from build123d import *

# Parameters (mm, degrees)
BOSS_EXTRU_1_DEPTH      = 6
BOSS_EXTRU_2_DEPTH      = 1.25
BOSS_EXTRU_2_DEPTH_BACK = 1.25
BOSS_EXTRU_3_DEPTH      = 1
ESQUISSE4_W             = 9.998484941
ESQUISSE4_H             = 1.4
BOSS_EXTRU_4_DEPTH      = 4.5
ESQUISSE6_W             = 1.25
ESQUISSE6_H             = 4.5
ENL_V_MAT_EXTRU_1_DEPTH = 0.7
CHANFREIN1_SIZE         = 0.7
BOSS_EXTRU_5_DEPTH      = 1.351515059
BOSS_EXTRU_6_DEPTH      = 1.35
ESQUISSE9_W             = 0.76
ESQUISSE9_H             = 0.76
BOSS_EXTRU_7_DEPTH      = 4
CHANFREIN2_SIZE         = 0.25
ENL_V_MAT_EXTRU_2_REACH = 11.014
ESQUISSE10_W            = 5
ESQUISSE10_H            = 3.75
CHANFREIN3_SIZE         = 0.25
ENL_V_MAT_EXTRU_3_REACH = 11.274
ESQUISSE11_W            = 5
ESQUISSE11_H            = 1.25


with BuildPart() as part:
    # Esquisse1 → Boss.-Extru.1 (new body)
    with BuildSketch(Plane.XY):
        Polygon((5, 0), (-5, 0), (-5, 5.5), (-3.33, 5.5), (-3.33, 4.5), (3.33, 4.5), (3.33, 5.5), (5, 5.5), align=None)
        Polygon((-4.5, 5), (-3.53, 5), (-3.53, 4), (3.53, 4), (3.53, 5), (4.5, 5), (4.5, 0.5), (-4.5, 0.5), align=None, mode=Mode.SUBTRACT)
    extrude(amount=BOSS_EXTRU_1_DEPTH)

    # Esquisse2 → Boss.-Extru.2 (add, two sides: drawn at the far end of the back side and taken through both)
    with BuildSketch(Plane(origin=(0, 0, 0), x_dir=(0, 0, -1), z_dir=(1, 0, 0)).offset(-BOSS_EXTRU_2_DEPTH_BACK)):
        Polygon((-1, 5.5), (-2.5, 4.5), (-0.9, 4.5), (-0.9, 5.5), align=None)
    extrude(amount=BOSS_EXTRU_2_DEPTH + BOSS_EXTRU_2_DEPTH_BACK)

    # Esquisse3 → Boss.-Extru.3 (add)
    with BuildSketch(Plane(origin=(0, 0, 0), x_dir=(-1, 0, 0), z_dir=(0, 0, -1))):
        Polygon((-3.33, 5.5), (-5, 5.5), (-5, 0), (5, 0), (5, 5.5), (3.33, 5.5), (3.33, 4.5), (-3.33, 4.5), align=None)
    extrude(amount=-BOSS_EXTRU_3_DEPTH)

    # Esquisse4 → Boss.-Extru.4 (add)
    with BuildSketch(Plane(origin=(0, 4.5, 0), x_dir=(1, 0, 0), z_dir=(0, 1, 0))):
        with Locations((-0.000757529, 0.7)):
            Rectangle(ESQUISSE4_W, ESQUISSE4_H)
    extrude(amount=-BOSS_EXTRU_4_DEPTH)

    # Esquisse6 → Enlèv. mat.-Extru.1 (cut)
    with BuildSketch(Plane(origin=(0, 0, -1.4), x_dir=(-1, 0, 0), z_dir=(0, 0, -1))):
        with Locations((-3.023484941, 2.25)):
            Rectangle(ESQUISSE6_W, ESQUISSE6_H)
        with Locations((1.008484941, 2.25)):
            Rectangle(ESQUISSE6_W, ESQUISSE6_H)
        with Locations((-1.008484941, 2.25)):
            Rectangle(ESQUISSE6_W, ESQUISSE6_H)
        with Locations((3.023484941, 2.25)):
            Rectangle(ESQUISSE6_W, ESQUISSE6_H)
    extrude(amount=-ENL_V_MAT_EXTRU_1_DEPTH, mode=Mode.SUBTRACT)

    # Chanfrein1
    chanfrein1_edges = [part.edges().sort_by_distance(p)[0] for p in [
        (3.023484941, 4.5, -0.7),
        (1.008484941, 4.5, -0.7),
        (-1.008484941, 4.5, -0.7),
        (-3.023484941, 4.5, -0.7),
    ]]
    chamfer(chanfrein1_edges, length=CHANFREIN1_SIZE - 0.0001)  # a hair under: the kernel refuses the full size

    # Esquisse7 → Boss.-Extru.5 (add)
    with BuildSketch(Plane.ZY.offset(5)):
        Polygon((-1.4, 0), (-3, 0), (-3, 0.75), (-1.4, 1.5), align=None)
    extrude(amount=-BOSS_EXTRU_5_DEPTH)

    # Esquisse8 → Boss.-Extru.6 (add)
    with BuildSketch(Plane(origin=(4.998484941, 0, 0), x_dir=(0, 0, -1), z_dir=(1, 0, 0))):
        Polygon((1.4, 0), (3, 0), (3, 0.75), (1.4, 1.5), align=None)
    extrude(amount=-BOSS_EXTRU_6_DEPTH)

    # Esquisse9 → Boss.-Extru.7 (add)
    with BuildSketch(Plane.XY.offset(1)):
        with Locations((-1.27, 2.38)):
            Rectangle(ESQUISSE9_W, ESQUISSE9_H)
        with Locations((3.81, 2.38)):
            Rectangle(ESQUISSE9_W, ESQUISSE9_H)
        with Locations((-3.81, 2.38)):
            Rectangle(ESQUISSE9_W, ESQUISSE9_H)
        with Locations((1.27, 2.38)):
            Rectangle(ESQUISSE9_W, ESQUISSE9_H)
    extrude(amount=BOSS_EXTRU_7_DEPTH)

    # Chanfrein2
    chanfrein2_edges = [part.edges().sort_by_distance(p)[0] for p in [
        (-1.65, 2.38, 5),
        (-1.27, 2, 5),
        (-0.89, 2.38, 5),
        (-1.27, 2.76, 5),
        (-3.43, 2.38, 5),
        (-3.81, 2.76, 5),
        (-4.19, 2.38, 5),
        (-3.81, 2, 5),
        (3.81, 2, 5),
        (4.19, 2.38, 5),
        (3.81, 2.76, 5),
        (3.43, 2.38, 5),
        (1.27, 2.76, 5),
        (0.89, 2.38, 5),
        (1.27, 2, 5),
        (1.65, 2.38, 5),
    ]]
    chamfer(chanfrein2_edges, length=CHANFREIN2_SIZE)

    # Esquisse10 → Enlèv. mat.-Extru.2 (cut, up to next)
    with BuildSketch(Plane(origin=(0, 4.5, 0), x_dir=(1, 0, 0), z_dir=(0, 1, 0)), mode=Mode.PRIVATE) as enl_v_mat_extru_2_sk1:
        with Locations((0, -4.375)):
            Rectangle(ESQUISSE10_W, ESQUISSE10_H)
    enl_v_mat_extru_2_tool1 = extrude(enl_v_mat_extru_2_sk1.sketch, amount=-ENL_V_MAT_EXTRU_2_REACH, mode=Mode.PRIVATE) & part.part
    add(enl_v_mat_extru_2_tool1.solids().sort_by_distance((0, 4.5, 4.375))[0], mode=Mode.SUBTRACT)

    # Chanfrein3
    chanfrein3_edges = [part.edges().sort_by_distance(p)[0] for p in [
        (2.5, 4.25, 6),
        (-2.5, 4.25, 6),
    ]]
    chamfer(chanfrein3_edges, length=CHANFREIN3_SIZE)

    # Esquisse11 → Enlèv. mat.-Extru.3 (cut, up to next)
    with BuildSketch(Plane(origin=(0, 0.5, 0), x_dir=(1, 0, 0), z_dir=(0, 1, 0)), mode=Mode.PRIVATE) as enl_v_mat_extru_3_sk1:
        with Locations((0, -5.625)):
            Rectangle(ESQUISSE11_W, ESQUISSE11_H)
    enl_v_mat_extru_3_tool1 = extrude(enl_v_mat_extru_3_sk1.sketch, amount=-ENL_V_MAT_EXTRU_3_REACH, mode=Mode.PRIVATE) & part.part
    add(enl_v_mat_extru_3_tool1.solids().sort_by_distance((0, 0.5, 5.625))[0], mode=Mode.SUBTRACT)


solid = part.part
Source: CAD feature listing. Evaluate the final solid. Frame: model axes, mm. A direction names the side the tool comes from. Round coordinates to 2 decimals unless told otherwise and drop trailing zeros. Loops run counter-clockwise (first coordinate to the right, second up) from the corner with the lowest first, then second, coordinate; pieces in that order, holes last. Notation, with made-up numbers: M -6.5,63 L 0.5,63 A23 cw 0.5,86 Z; hole C -31.75,80.25 d8. An arc over 180 degrees is marked long. Return JSON: item names as keys, results as strings. Group by question number.
1. Reachability of faces 4 (the face through (3.33, 5, 3)), 5 (the face through (5, 3, 3)), 6 (the face through (-3, 2, -0.7)), 7 (the face through (-4.5, 3, 3)), 8 (the face through (-0.018, 5.007, 1.74)) from +Z, -Z, +X, -X, +Y, -Y: full face, straight path, thin tool, end or side. Return the list, or none.
2. Material intervals for line 1 along X through (y, z) = (2.4, 1.5); line 2 along X through (y, z) = (4.9, 4.5); line 3 along X through (y, z) = (2.4, -1.25), sorted ascending. Write a range as from..to.
3. Mould query, pull axis Y, two halves, no side actions, for faces 1 (the face through (-4, 5, 0)), 2 (the face through (-4.33, 1.12, -2.21)), 3 (the face through (-4, 5, 3)). Classes: released by +Y, released by -Y, zero draft, split by the parting line, or undercut.
4. Pin query (flat end, axial travel): pin 1 (1 mm diameter, centred on x = -1, y = 4, fed in from +Z); pin 2 (1.5 mm diameter, centred on x = 1, z = -0.5, fed in from +Y); pin 3 (3 mm diameter, centred on x = -1, y = 2, fed in from +Z). Return the tip coordinate at first contact, or that it passes through.
5. Section query B-B on x = -3. Output: boundary loops of the cut face in (y, z), and give its area (3 significant figures).
6. Section query A-A on y = 5.2. Output: boundary loops of the cut face in (x, z).
7. Section query C-C on z = 2.75. State how many separate pieces and enclosed holes the cut face has, and give its area (3 significant figures).
8. Section query D-D on z = -0.5. Output: boundary loops of the cut face in (x, y).
Checks:
{
 "1": {"face 4": "+Z, -Z, +Y", "face 5": "+Z, -Z, +X, +Y, -Y", "face 6": "-Z, +Y, -Y", "face 7": "+Z", "face 8": "+Z, +Y"},
 "2": {"line 1": "x = -5..-4.5, -4.19..-3.43, -1.65..-0.89, 0.89..1.65, 3.43..4.19, 4.5..5", "line 2": "x = -5..-4.5, -3.53..-3.33, 3.33..3.53, 4.5..5", "line 3": "x = -5..-3.65, -2.4..-1.63, -0.38..0.38, 1.63..2.4, 3.65..5"},
 "3": {"face 1": "zero draft", "face 2": "released by +Y", "face 3": "undercut"},
 "4": {"pin 1": "stops at z = 2.5", "pin 2": "stops at y = 4.5", "pin 3": "stops at z = 5"},
 "5": {"outline": "M 0,-0.7 L 3.8,-0.7 L 4.5,0 L 4.5,6 L 4,6 L 4,1 L 0.5,1 L 0.5,6 L 0,6 Z", "area": "12.4 mm²"},
 "6": {"outline": "M -5,0 L -3.33,0 L -3.33,6 L -5,6 Z; M -1.25,0.9 L 1.25,0.9 L 1.25,1.45 L -1.25,1.45 Z; M 3.33,0 L 5,0 L 5,6 L 3.33,6 Z"},
 "7": {"separate pieces": "5", "enclosed holes": "0", "area": "14.7 mm²"},
 "8": {"outline": "M -5,0 L 5,0 L 5,4.5 L 3.65,4.5 L 3.65,4 L 2.4,4 L 2.4,4.5 L 1.63,4.5 L 1.63,4 L 0.38,4 L 0.38,4.5 L -0.38,4.5 L -0.38,4 L -1.63,4 L -1.63,4.5 L -2.4,4.5 L -2.4,4 L -3.65,4 L -3.65,4.5 L -5,4.5 Z"}
}
